CAD build for the part. Positions are in the model's coordinates, mm. Face numbers are marked on the shaded views. Coordinates: 2 decimals unless noted, no trailing zeros. Write each loop counter-clockwise with the first axis right and the second up, starting at its lowest first coordinate (ties: lowest second). Pieces come first, ordered by that corner, then holes. Notation, with made-up numbers: (77, 4) -> (82, 4) arc R12 ccw to (82, 15) -> close; hole circle Ø3 at (-12.75, -4). An arc over 180 degrees is marked (long way). Answer as CSV lines item,"result". Start each with the question number.
```python
from build123d import *

# Parameters (mm, degrees)
SKETCH1_R           = 60.96
BOSS_EXTRUDE1_DEPTH = 19.05
FILLET1_R           = 2.54
SKETCH2_R           = 4
CUT_EXTRUDE1_DEPTH  = 6.35
SKETCH4_R           = 25.019
CUT_EXTRUDE3_DEPTH  = 89.290122324
SKETCH5_R           = 3.175
CUT_EXTRUDE4_DEPTH  = 89.290122324
CIRPATTERN2_COUNT   = 8
SKETCH6_R           = 25.019
SKETCH6_R_2         = 4.09575
BOSS_EXTRUDE2_DEPTH = 3.175


with BuildPart() as part:
    # Sketch1 → Boss-Extrude1 (new body)
    with BuildSketch(Plane(origin=(0, 0, 0), x_dir=(0, 0, -1), z_dir=(1, 0, 0))):
        with Locations(Location((0, 0, 0), (0, 0, 180))):
            Circle(SKETCH1_R)
    extrude(amount=BOSS_EXTRUDE1_DEPTH)

    # Fillet1
    fillet1_edges = [part.edges().sort_by_distance(p)[0] for p in [
        (19.05, 0, -60.96),
    ]]
    fillet(fillet1_edges, radius=FILLET1_R)

    # Sketch2 → Cut-Extrude1 (cut)
    with BuildSketch(Plane(origin=(19.05, 0, 0), x_dir=(0, 0, -1), z_dir=(1, 0, 0))):
        Circle(SKETCH2_R)
    extrude(amount=-CUT_EXTRUDE1_DEPTH, mode=Mode.SUBTRACT)

    # Sketch4 → Cut-Extrude3 (cut, through all)
    with BuildSketch(Plane(origin=(19.05, 0, 0), x_dir=(0, 0, -1), z_dir=(1, 0, 0))):
        Circle(SKETCH4_R)
    extrude(amount=-CUT_EXTRUDE3_DEPTH, mode=Mode.SUBTRACT)

    # Sketch5 → Cut-Extrude4 (cut, through all)
    with BuildSketch(Plane.ZY):
        with Locations((-35.91734849, 35.383889532)):
            Circle(SKETCH5_R)
    cut_extrude4 = extrude(amount=-CUT_EXTRUDE4_DEPTH, mode=Mode.SUBTRACT)

    # CirPattern2: Cut-Extrude4 ×8 about axis, 1 skipped
    cirpattern2_axis = Axis((0, 0, 0), (1, 0, 0))
    add([cut_extrude4.rotate(cirpattern2_axis, i * 360 / CIRPATTERN2_COUNT) for i in range(1, CIRPATTERN2_COUNT) if i not in (7,)], mode=Mode.SUBTRACT)

    # Sketch6 → Boss-Extrude2 (add)
    with BuildSketch(Plane(origin=(19.05, 0, 0), x_dir=(0, 0, -1), z_dir=(1, 0, 0))):
        Circle(SKETCH6_R)
        Circle(SKETCH6_R_2, mode=Mode.SUBTRACT)
    extrude(amount=-BOSS_EXTRUDE2_DEPTH)


solid = part.part
```
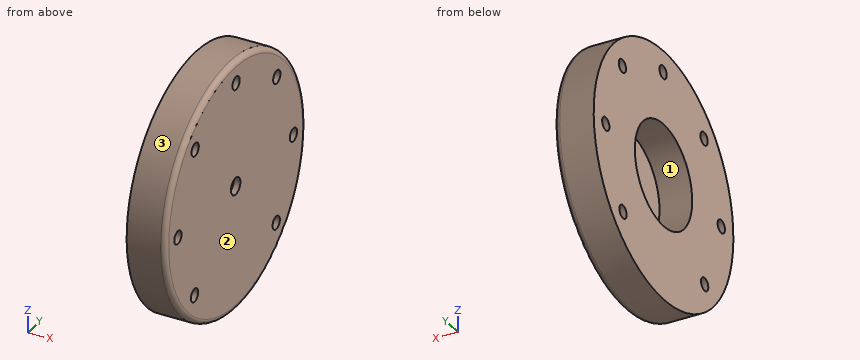
1. Mould opens along Y. For the marked faces 1, 2 and 3 say: pulls with the +Y half, pulls with the -Y half, needs draft (parallel to the pull), parting line crosses it, or undercut.
2. Flat gauge pins, fed straight in: P1, Ø5, axis at x = 4.5, y = 46, coming from the -Z side; P2, Ø1.5, axis at x = 3.5, y = -43.5, coming from the -Z side; P3, Ø4, axis at y = 50.42, z = -0.38, coming from the +X side; P4, Ø8, axis at x = 16.5, z = 2.5, coming from the +Y side. Where does each tip first touch, or does it go through?
3. Cut at A-A (y = 0). Give the cut face in (x, z) (3 decimals).
4. Cut at B-B (x = 14.25). Count the separate pieces of the cut face and the enclosed holes in it, then the cut area to 3 significant figures.
5. Cut at C-C (z = 0). Give the cut face in (x, y) (3 decimals).
6. Wall check: line 1 (Y direction, x = 8.25, z = 0); line 2 (Y direction, x = 16.7, z = 0); line 3 (Z direction, x = 17, y = 37). Give the ranges that are in metal, low to high.
Geometry check:
1,face 1,"undercut"
1,face 2,"needs draft"
1,face 3,"parting line crosses it"
2,P1,"z = -42.71"
2,P2,"z = -43.46"
2,P3,"through"
2,P4,"y = 60.96"
3,outline,"(0, -60.96) -> (16.51, -60.96) arc R2.54 ccw to (19.05, -58.42) -> (19.05, -4.096) -> (15.875, -4.096) -> (15.875, -25.019) -> (0, -25.019) -> close; (0, 25.019) -> (15.875, 25.019) -> (15.875, 4.096) -> (19.05, 4.096) -> (19.05, 47.265) -> (0, 47.265) -> close; (0, 53.57) -> (19.05, 53.57) -> (19.05, 58.42) arc R2.54 ccw to (16.51, 60.96) -> (0, 60.96) -> close"
4,separate pieces,"1"
4,enclosed holes,"8"
4,area,"9,490 mm²"
5,outline,"(0, -60.96) -> (16.51, -60.96) arc R2.54 ccw to (19.05, -58.42) -> (19.05, -53.57) -> (0, -53.57) -> close; (0, -47.265) -> (19.05, -47.265) -> (19.05, -4.096) -> (15.875, -4.096) -> (15.875, -25.019) -> (0, -25.019) -> close; (0, 25.019) -> (15.875, 25.019) -> (15.875, 4.096) -> (19.05, 4.096) -> (19.05, 47.265) -> (0, 47.265) -> close; (0, 53.57) -> (19.05, 53.57) -> (19.05, 58.42) arc R2.54 ccw to (16.51, 60.96) -> (0, 60.96) -> close"
6,line 1,"-60.96 to -53.57, -47.27 to -25.02, 25.02 to 47.27, 53.57 to 60.96"
6,line 2,"-60.95 to -53.57, -47.27 to -4.1, 4.1 to 47.27, 53.57 to 60.95"
6,line 3,"-48.39 to -38.65, -33.18 to 32.4, 38.37 to 48.39"
